For this review, take the finished solid that the model builds, in its own axes (mm). A direction names the side the tool comes from. Round coordinates to 2 decimals unless told otherwise and drop trailing zeros. Order: outer loops, then holes, each group sorted by start corner. A loop starts at its lowest first (then second) coordinate and runs counter-clockwise, first axis right, second up.
```python
from build123d import *

# Parameters (mm, degrees)
SKETCH1_W           = 88
SKETCH1_H           = 37
SKETCH1_R           = 1.6
BOSS_EXTRUDE1_DEPTH = 5
FILLET1_R           = 5
CHAMFER2_SIZE       = 1.5
SKETCH2_R           = 1.25
CUT_EXTRUDE1_DEPTH  = 10


with BuildPart() as part:
    # Sketch1 → Boss-Extrude1 (new body)
    with BuildSketch(Plane.YZ):
        Rectangle(SKETCH1_W, SKETCH1_H)
        with Locations(Location((-41.5, -15.5, 0), (0, 0, 270))):
            Circle(SKETCH1_R, mode=Mode.SUBTRACT)
        with Locations(Location((-41.5, -3, 0), (0, 0, 270))):
            Circle(SKETCH1_R, mode=Mode.SUBTRACT)
        with Locations(Location((41.5, -15.5, 0), (0, 0, 90))):
            Circle(SKETCH1_R, mode=Mode.SUBTRACT)
        with Locations(Location((-26, 14, 0), (0, 0, 270))):
            Circle(SKETCH1_R, mode=Mode.SUBTRACT)
        with Locations(Location((-26, -12, 0), (0, 0, 270))):
            Circle(SKETCH1_R, mode=Mode.SUBTRACT)
        with Locations(Location((41.5, -0.5, 0), (0, 0, 270))):
            Circle(SKETCH1_R, mode=Mode.SUBTRACT)
        with BuildLine():
            Line((-24, -8.2), (-24, 11.8))
            ThreePointArc((-24, 11.8), (-22.86444197, 13.331108636), (-21.069632929, 12.688888889))
            ThreePointArc((-21.069632929, 12.688888889), (-20.349483132, 12.036165793), (-19.406674091, 11.8))
            Line((-19.406674091, 11.8), (26.806674091, 11.8))
            ThreePointArc((26.806674091, 11.8), (27.749483132, 12.036165793), (28.469632929, 12.688888889))
            ThreePointArc((28.469632929, 12.688888889), (30.26444197, 13.331108636), (31.4, 11.8))
            Line((31.4, 11.8), (31.4, -8.2))
            ThreePointArc((31.4, -8.2), (30.26444197, -9.731108636), (28.469632929, -9.088888889))
            ThreePointArc((28.469632929, -9.088888889), (27.749483132, -8.436165793), (26.806674091, -8.2))
            Line((26.806674091, -8.2), (-19.406674091, -8.2))
            ThreePointArc((-19.406674091, -8.2), (-20.349483132, -8.436165793), (-21.069632929, -9.088888889))
            ThreePointArc((-21.069632929, -9.088888889), (-22.86444197, -9.731108636), (-24, -8.2))
        make_face(mode=Mode.SUBTRACT)
    extrude(amount=BOSS_EXTRUDE1_DEPTH)

    # Fillet1
    fillet1_edges = [part.edges().sort_by_distance(p)[0] for p in [
        (2.5, -44, 18.5),
        (2.5, 44, 18.5),
    ]]
    fillet(fillet1_edges, radius=FILLET1_R)

    # Chamfer2
    # the kernel refuses this chamfer: 1.5 mm, written as the material it takes off along each edge
    with BuildSketch(Plane(origin=(5, -41.5, -15.5), x_dir=(0, 0, -1), z_dir=(0, -1, 0))) as chamfer2_piece_1:
        Polygon((1.6 + CHAMFER2_SIZE, 0), (1.6, -CHAMFER2_SIZE), (1.6, 0), align=None)
    revolve(axis=Axis((5, -41.5, -15.5), (1, 0, 0)), mode=Mode.SUBTRACT)
    with BuildSketch(Plane(origin=(5, -41.5, -3), x_dir=(0, 0, -1), z_dir=(0, -1, 0))) as chamfer2_piece_2:
        Polygon((1.6 + CHAMFER2_SIZE, 0), (1.6, -CHAMFER2_SIZE), (1.6, 0), align=None)
    revolve(axis=Axis((5, -41.5, -3), (1, 0, 0)), mode=Mode.SUBTRACT)
    with BuildSketch(Plane(origin=(5, 41.5, -0.5), x_dir=(0, 0, -1), z_dir=(0, -1, 0))) as chamfer2_piece_3:
        Polygon((1.6 + CHAMFER2_SIZE, 0), (1.6, -CHAMFER2_SIZE), (1.6, 0), align=None)
    revolve(axis=Axis((5, 41.5, -0.5), (1, 0, 0)), mode=Mode.SUBTRACT)
    with BuildSketch(Plane(origin=(5, 41.5, -15.5), x_dir=(0, 0, 1), z_dir=(0, 1, 0))) as chamfer2_piece_4:
        Polygon((1.6 + CHAMFER2_SIZE, 0), (1.6, -CHAMFER2_SIZE), (1.6, 0), align=None)
    revolve(axis=Axis((5, 41.5, -15.5), (1, 0, 0)), mode=Mode.SUBTRACT)
    with BuildSketch(Plane(origin=(5, -26, 14), x_dir=(0, 0, -1), z_dir=(0, -1, 0))) as chamfer2_piece_5:
        Polygon((1.6 + CHAMFER2_SIZE, 0), (1.6, -CHAMFER2_SIZE), (1.6, 0), align=None)
    revolve(axis=Axis((5, -26, 14), (1, 0, 0)), mode=Mode.SUBTRACT)
    with BuildSketch(Plane(origin=(5, -26, -12), x_dir=(0, 0, -1), z_dir=(0, -1, 0))) as chamfer2_piece_6:
        Polygon((1.6 + CHAMFER2_SIZE, 0), (1.6, -CHAMFER2_SIZE), (1.6, 0), align=None)
    revolve(axis=Axis((5, -26, -12), (1, 0, 0)), mode=Mode.SUBTRACT)

    # Sketch2 → Cut-Extrude1 (cut)
    with BuildSketch(Plane.YZ.offset(5)):
        with Locations(Location((-36.826603685, -0.023130638, 0), (0, 0, 270))):
            Circle(SKETCH2_R)
        with Locations(Location((-33.167413509, -14.120748425, 0), (0, 0, 270))):
            Circle(SKETCH2_R)
        with Locations(Location((33.182572395, -14.077498807, 0), (0, 0, 270))):
            Circle(SKETCH2_R)
    extrude(amount=-CUT_EXTRUDE1_DEPTH, mode=Mode.SUBTRACT)


solid = part.part
```
Q1. Take a section at A-A, the plane y = 12. State the section outline as (x, z) points, plus the area to 3 significant figures.
Q2. Take a section at D-D, the plane y = 41.5. State the section outline as (x, z) points, plus the area to 3 significant figures.
Q3. Wall thickness on line 1 (Y direction, x = 2.45, z = -3); line 2 (Y direction, x = 1.8, z = -12); line 3 (Z direction, x = 1.85, y = -4): over which ranges is each line inside the solid? List them lowest first.
Q4. Take a section at B-B, the plane y = -26. State the section outline as (x, z) points, plus the area to 4 significant figures.
Q5. Tool access review of faces 1 (the face through (5, -1, 13)), 2 (the face through (2.465, 30.292, -9.723)): name each direction out of +Z, -Z, +X, -X, +Y, -Y from which nothing blocks a thin tool from reaching the whole face with its end or side.
Q6. Clearance check with flat-ended pins moving along their axes: pin 1 (1.9 mm diameter, centred on y = -41.5, z = -3, fed in from +X); pin 2 (4 mm diameter, centred on y = -26, z = -12, fed in from +X). State where each tip first meets the part, or that it passes through.
Q7. Mouldability with a two-part tool opening along Z and no side actions: class faces 3 (the face through (2.54, -42.57, 17)), 4 (the face through (3.739, -39.676, -2.761)), 5 (the face through (2, -44, -3)), 6 (the face through (2, -1, -18.5)) as +Z half, -Z half, draft (parallel to the pull), parting line (faces both ways), or undercut.
Q8. Take a section at C-C, the plane x = 1.75. Count the separate pieces of the cut face and the enclosed holes in it, plus the area to 3 significant figures.
Working result:
1. outline: (0, -18.5) - (5, -18.5) - (5, -8.2) - (0, -8.2) - close; (0, 11.8) - (5, 11.8) - (5, 18.5) - (0, 18.5) - close
1. area: 85.0 mm2
2. outline: (0, -18.5) - (4.9, -18.5) - (3.5, -17.1) - (0, -17.1) - close; (0, -13.9) - (3.5, -13.9) - (5, -12.4) - (5, -3.6) - (3.5, -2.1) - (0, -2.1) - close; (0, 1.1) - (3.5, 1.1) - (5, 2.6) - (5, 17.83) - (0, 17.83) - close
2. area: 145 mm2
3. line 1: y = -44 to -43.1, -39.9 to -24, 31.4 to 44
3. line 2: y = -44 to -27.6, -24.4 to 44
3. line 3: z = -18.5 to -8.2, 11.8 to 18.5
4. outline: (0, -18.5) - (5, -18.5) - (5, -15.1) - (3.5, -13.6) - (0, -13.6) - close; (0, -10.4) - (3.5, -10.4) - (5, -8.9) - (5, 10.9) - (3.5, 12.4) - (0, 12.4) - close; (0, 15.6) - (3.5, 15.6) - (5, 17.1) - (5, 18.5) - (0, 18.5) - close
4. area: 148.5 mm2
5. face 1: +Z, -Z, +X, +Y, -Y
5. face 2: +X, -X
6. pin 1: passes through
6. pin 2: stops at x = 3.9
7. face 3: +Z half
7. face 4: undercut
7. face 5: draft
7. face 6: -Z half
8. separate pieces: 1
8. enclosed holes: 10
8. area: 2,060 mm2
